Geometry: see drawing. Coordinates: mm, zero at the bounding-box minimum. Coordinates: 2 decimals unless noted, no trailing zeros. Write each loop counter-clockwise with the first axis right and the second up, starting at its lowest first coordinate (ties: lowest second). Pieces come first, ordered by that corner, then holes.
1) Line query: L1, parallel to Y at x = 15.75, z = 0.35; L2, parallel to Y at x = 15, z = 0.8; L3, parallel to X at y = 31.5, z = 0.4. Output: solid intervals per line, ascending.
2) Section query B-B (x = 15.75). Output: boundary loops of the cut face in (y, z).
3) Pin query (flat end, axial travel): pin 1 Ø4 at (x, y) = (15.75, 30) entering from -Z. Return the tip coordinate at first contact, or that it passes through.
4) Section query A-A (y = 30). Output: boundary loops of the cut face in (x, z).
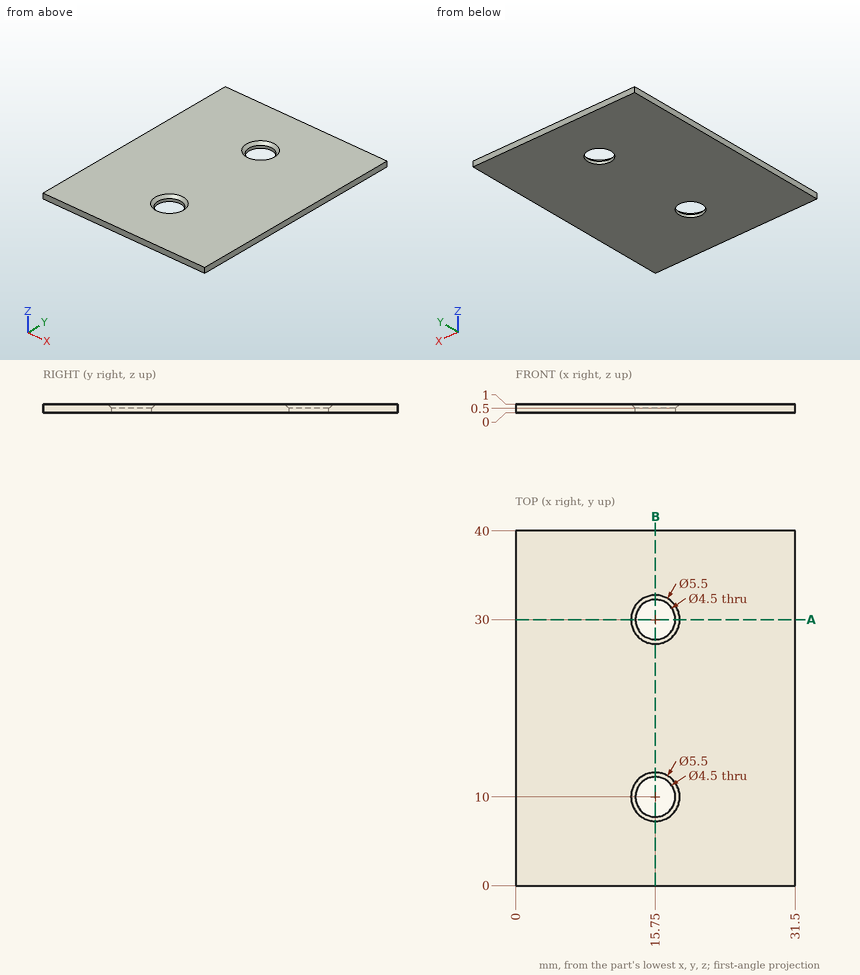
Answer:
1. L1: y = 0 to 7.75, 12.25 to 27.75, 32.25 to 40
1. L2: y = 0 to 7.56, 12.44 to 27.56, 32.44 to 40
1. L3: x = 0 to 14.07, 17.43 to 31.5
2. outline: (0, 0) - (7.75, 0) - (7.75, 0.5) - (7.25, 1) - (0, 1) - close; (12.25, 0) - (27.75, 0) - (27.75, 0.5) - (27.25, 1) - (12.75, 1) - (12.25, 0.5) - close; (32.25, 0) - (40, 0) - (40, 1) - (32.75, 1) - (32.25, 0.5) - close
3. pin 1: passes through
4. outline: (0, 0) - (13.5, 0) - (13.5, 0.5) - (13, 1) - (0, 1) - close; (18, 0) - (31.5, 0) - (31.5, 1) - (18.5, 1) - (18, 0.5) - close
